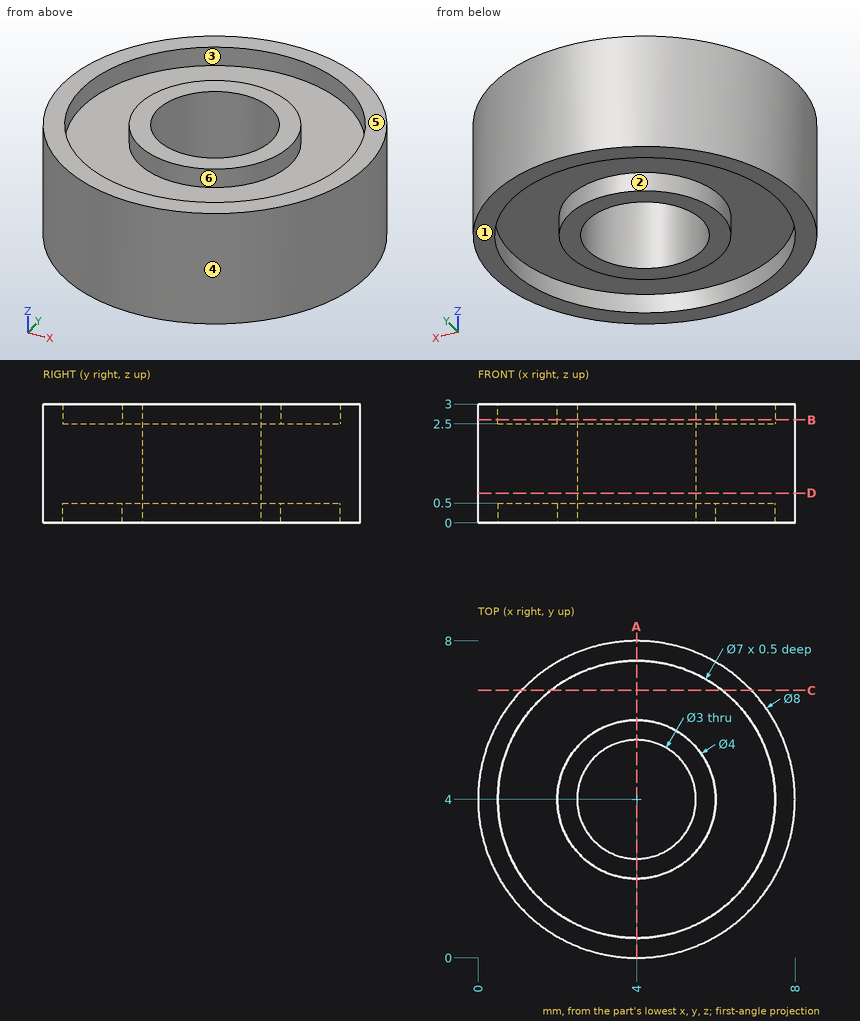
Design review of the part shown in the three views and the two pictorial views. Dimensions are in mm from the part's minimum x, y and z. A direction names the side the tool comes from. Give positions to 0.01 mm unless a question says otherwise; leave off trailing zeros. Order: outer loops, then holes, each group sorted by start corner. A loop starts at its lowest first (then second) coordinate and runs counter-clockwise, first axis right, second up. Notation, with made-up numbers: (5, 29) -> (23, 29) arc R22 ccw to (23, 44) -> close; hole circle Ø5 at (-2, 1). An arc over 180 degrees is marked (long way). Write each question's results on one line, items separated by ' | '. Start each with the question number.
Q1. Wall thickness on L1, parallel to Y at x = 4, z = 2.8; L2, parallel to Y at x = 4, z = 1.9; L3, parallel to Z at x = 6.25, y = 5: over which ranges is each line inside the solid? List them lowest first. Write a range as from..to.
Q2. Add section C-C on y = 6.75. Give the boundary of the cut face in (x, z).
Q3. Machinability: for the marked faces 1, 2 and 3, which of the approach directions +Z, -Z, +X, -X, +Y, -Y give a long, thin tool a straight path to every point of the face, cutting with its end or side? Answer none if there is none.
Q4. Add section A-A on x = 4. Give the boundary of the cut face in (y, z), and give its area (3 significant figures).
Q5. Add section B-B on z = 2.6. Give the boundary of the cut face in (x, y).
Q6. Add section D-D on z = 0.75. Give the boundary of the cut face in (x, y), and give its area (3 significant figures).
Q7. Mouldability with a two-part tool opening along X and no side actions: class the marked faces 4, 5 and 6 as +X half, -X half, draft (parallel to the pull), parting line (faces both ways), or undercut.
Q8. For pin 1 (2 mm diameter, centred on x = 4, y = 5.5, fed in from -Z); pin 2 (1.8 mm diameter, centred on x = 4, y = 4, fed in from +Z), all flat-tipped, find the tip position at first contact; note any pin that passes through.
Found:
1) L1: y = 0..0.5, 2..2.5, 5.5..6, 7.5..8 | L2: y = 0..2.5, 5.5..8 | L3: z = 0.5..2.5
2) outline: (1.1, 0) -> (1.83, 0) -> (1.83, 0.5) -> (6.17, 0.5) -> (6.17, 0) -> (6.9, 0) -> (6.9, 3) -> (6.17, 3) -> (6.17, 2.5) -> (1.83, 2.5) -> (1.83, 3) -> (1.1, 3) -> close
3) face 1: -Z, +X, -X, +Y, -Y | face 2: -Z | face 3: +Z
4) outline: (0, 0) -> (0.5, 0) -> (0.5, 0.5) -> (2, 0.5) -> (2, 0) -> (2.5, 0) -> (2.5, 3) -> (2, 3) -> (2, 2.5) -> (0.5, 2.5) -> (0.5, 3) -> (0, 3) -> close; (5.5, 0) -> (6, 0) -> (6, 0.5) -> (7.5, 0.5) -> (7.5, 0) -> (8, 0) -> (8, 3) -> (7.5, 3) -> (7.5, 2.5) -> (6, 2.5) -> (6, 3) -> (5.5, 3) -> close | area: 12.0 mm2
5) outline: circle Ø8 at (4, 4); circle Ø4 at (4, 4); hole circle Ø7 at (4, 4); hole circle Ø3 at (4, 4)
6) outline: circle Ø8 at (4, 4); hole circle Ø3 at (4, 4) | area: 43.2 mm2
7) face 4: parting line | face 5: draft | face 6: undercut
8) pin 1: stops at z = 0 | pin 2: passes through
